Autodesk Inventor part; units mm, degrees
ref_plane "YZ Plane" through (0, 0, 0) normal (1, 0, 0) x (0, 1, 0)
ref_plane "XZ Plane" through (0, 0, 0) normal (0, 1, 0) x (-1, 0, 0)
ref_plane "XY Plane" through (0, 0, 0) normal (0, 0, 1) x (1, 0, 0)
sketch "Sketch1" plane through (0, 0, 0) normal (0, 1, 0) x (-1, 0, 0)
  circle A0 centre (0, 0) radius 73.025
  line L0 (0, 0) -> (0, -73.025) construction
  line L1 (0, 0) -> (-12.6807, -71.9156)
  line L2 (0, 0) -> (12.6807, -71.9156)
  line L3 (0, 0) -> (72.3143, -10.1631)
  line L4 (0, 0) -> (64.4772, -34.2832)
  line L5 (0, 0) -> (32.0121, 65.6344)
  line L6 (0, 0) -> (52.5298, 50.7274)
  line L7 (0, 0) -> (-52.5298, 50.7274)
  line L8 (0, 0) -> (-32.0121, 65.6344)
  line L9 (0, 0) -> (-64.4772, -34.2832)
  line L10 (0, 0) -> (-72.3143, -10.1631)
  circle A1 centre (0, 0) radius 69.85
  arc A2 (4.7597, -69.6876) -> (-4.7597, -69.6876) centre (0, -69.85) ccw
  arc A3 (67.7477, -17.0079) -> (64.806, -26.0614) centre (66.4313, -21.5848) ccw
  arc A4 (37.1107, 59.1762) -> (44.8121, 53.5808) centre (41.0568, 56.5098) ccw
  arc A5 (-44.8121, 53.5808) -> (-37.1107, 59.1762) centre (-41.0568, 56.5098) ccw
  arc A6 (-64.806, -26.0614) -> (-67.7477, -17.0079) centre (-66.4313, -21.5848) ccw
  point P0 (61.6739, -32.7926)
  point P1 (69.1702, -9.7212)
  point P2 (50.2459, 48.5219)
  point P3 (30.6202, 62.7808)
  point P4 (-30.6202, 62.7808)
  point P5 (-50.2459, 48.5219)
  point P6 (-69.1702, -9.7212)
  point P7 (-61.6739, -32.7926)
  point P8 (-12.1293, -68.7888)
  point P9 (12.1293, -68.7888)
  point P10 (64.806, -26.0614)
  point P11 (67.7477, -17.0079)
  point P12 (44.8121, 53.5808)
  point P13 (37.1107, 59.1762)
  point P14 (-37.1107, 59.1762)
  point P15 (-67.7477, -17.0079)
  dimension "d0" = 146.05
  dimension "d1" = 10
  dimension "d4" = 360
  dimension "d6" = 3.175
  dimension "d10" = 9.525
  dimension "d13" = 360
extrude "Extrusion1" add sketch "Sketch1" along normal blind 3.175 contours A0 L3 A1 L6 | L5 A1 L8 A0 | A1 L3 L6 | L6 L5 A1 A4 | A0 L2 A1 L4 | A1 A3 L4 L3 | L5 L8 A1 | L2 A1 A2 L1 | L4 A1 L2 | L10 A1 L7 | L7 A1 A5 L8 | L1 A1 L9 | L9 A1 A6 L10 | A0 L1 A1 L2 | L7 A1 L10 A0 | L1 A0 L9 A1 | A2 A1
fillet "Fillet1" radius 1.5875 24 edges at (30.6202, 1.5875, 62.7808) (32.0121, 1.5875, 65.6344) (-30.6202, 1.5875, 62.7808) (-32.0121, 1.5875, 65.6344) (-52.5298, 1.5875, 50.7274) (-50.2459, 1.5875, 48.5219) (52.5298, 1.5875, 50.7274) (50.2459, 1.5875, 48.5219) (64.4772, 1.5875, -34.2832) (61.6739, 1.5875, -32.7926) (72.3143, 1.5875, -10.1631) (69.1702, 1.5875, -9.7212) (-72.3143, 1.5875, -10.1631) (-69.1702, 1.5875, -9.7212) (-64.4772, 1.5875, -34.2832) (-61.6739, 1.5875, -32.7926) (37.1107, 1.5875, 59.1762) (44.8121, 1.5875, 53.5808) (-44.8121, 1.5875, 53.5808) (-37.1107, 1.5875, 59.1762) (-64.806, 1.5875, -26.0614) (-67.7477, 1.5875, -17.0079) (67.7477, 1.5875, -17.0079) (64.806, 1.5875, -26.0614)
sketch "Sketch5" plane through (0, 3.175, 0) normal (0, 1, 0) x (1, 0, 0)
  line L0 (0, 0) -> (0, 65.0875) construction
  circle A0 centre (0, 50.8) radius 22.225 construction
  arc A1 (63.6995, 35.7075) -> (-63.6995, 35.7075) centre (0, 0) ccw
  circle A2 centre (0, 50.8) radius 12.5 construction
  circle A3 centre (-24.6062, 60.325) radius 1.7526
  circle A4 centre (-24.6062, 60.325) radius 3.175 construction
  circle A5 centre (-22.225, 34.925) radius 3.175 construction
  circle A6 centre (-22.225, 34.925) radius 1.7526
  circle A7 centre (24.6062, 60.325) radius 1.7526 construction
  circle A8 centre (24.6062, 60.325) radius 3.175 construction
  circle A9 centre (22.225, 34.925) radius 3.175 construction
  circle A10 centre (22.225, 34.925) radius 1.7526 construction
  arc A11 (-62.3874, 31.414) -> (-64.248, 27.4085) centre (0, 0) ccw
  arc A12 (63.6995, 35.7075) -> (-63.6995, 35.7075) centre (0, 0) ccw
  line L1 (-28.4451, 67.2572) -> (-25.3861, 34.6286) construction
  line L2 (-22.7046, 31.7864) -> (-3.3572, 28.83) construction
  line L3 (28.4451, 67.2572) -> (25.3861, 34.6286) construction
  line L4 (22.7046, 31.7864) -> (3.3572, 28.83) construction
  circle A13 centre (0, 50.8) radius 6.35 construction
  circle A14 centre (0, 0) radius 73.025
  line L5 (0, 50.8) -> (-8.8388, 59.6388) construction
  circle A15 centre (0, 50.8) radius 9.5 construction
  line L6 (0, 50.8) -> (6.7175, 57.5175) construction
  circle A16 centre (-8.8388, 59.6388) radius 1.5 construction
  circle A17 centre (6.7175, 57.5175) radius 1.5 construction
  circle A18 centre (8.8388, 41.9612) radius 1.5 construction
  circle A19 centre (-6.7175, 44.0825) radius 1.5 construction
  line L7 (-24.6062, 60.325) -> (-22.225, 34.925) construction
  line L8 (-27.7674, 60.0286) -> (-25.3861, 34.6286)
  line L9 (-19.0639, 35.2214) -> (-21.4451, 60.6214)
  arc A20 (-21.4451, 60.6214) -> (-27.7674, 60.0286) centre (-24.6062, 60.325) ccw
  arc A21 (-25.3861, 34.6286) -> (-19.0639, 35.2214) centre (-22.225, 34.925) ccw
  circle A22 centre (-22.225, 34.925) radius 4.7625 construction
  circle A23 centre (-24.6062, 60.325) radius 4.7625 construction
  line L10 (-21.7805, 30.1833) -> (-25.0508, 65.0667) construction
  line L11 (-18.6193, 30.4796) -> (-21.8896, 65.3631)
  line L12 (-28.2119, 64.7704) -> (-24.9416, 29.8869)
  arc A24 (-24.9416, 29.8869) -> (-18.6193, 30.4796) centre (-21.7805, 30.1833) ccw
  arc A25 (-21.8896, 65.3631) -> (-28.2119, 64.7704) centre (-25.0508, 65.0667) ccw
  point P0 (-63.6995, 35.7075)
  point P1 (-23.4156, 47.625)
  point P2 (-63.6995, 35.7075)
  point P3 (-23.4156, 47.625)
  point P4 (-28.3025, 67.3173)
  point P5 (-23.3151, 69.203)
  dimension "d39" = 25
  dimension "d40" = 44.45
  dimension "d78" = 19
  dimension "d100" = 9.525
  dimension "d101" = 9.525
  dimension "d41" = 3.5052
  dimension "d42" = 6.35
  dimension "d43" = 9.525
  dimension "d44" = 24.6062
  dimension "d45" = 6.35
  dimension "d46" = 3.5052
  dimension "d47" = 15.875
  dimension "d48" = 22.225
  dimension "d68" = 12.7
  dimension "d77" = 315
  dimension "d79" = 3
  dimension "d80" = 3
  dimension "d83" = 360
  dimension "d102" = 6.35
extrude "Extrusion3" cut sketch "Sketch5" against normal blind 25.4
chamfer "Chamfer2" distance 1.524 angle 41 2 edges at (-23.9776, 3.175, -34.925) (-26.3589, 3.175, -60.325)
equation "\"d45\" = d42"
equation "\"d46\" = d41"
properties part number "Top Plate" material "UHMW, White"
Read the model definition and answer for the solid it produces. Units are mm, in the model's axes. Give positions to 0.01 mm unless a question says otherwise; leave off trailing zeros. Write each loop counter-clockwise with the first axis right and the second up, starting at its lowest first coordinate (ties: lowest second). Pieces come first, ordered by that corner, then holes. Notation, with made-up numbers: (58.25, -24.75) -> (88.25, -24.75) arc R23 ccw to (88.25, -15.75) -> close; hole circle Ø10 at (52.5, -10.75). An arc over 180 degrees is marked (long way). Answer in a Markdown table with one row per item.
1) This flat-tipped pin is pushed along its axis until it touches: pin 1 Ø5.5 at (x, z) = (-22.225, -34.925) entering from -Y. Where does it stop, or does it pass through?
Results list:
| item | result |
|---|---|
| pin 1 | y = 0 |
2) Section B-B on z = -44 is taken. Give the vertices of the cut face in (x, y) (3 decimals), plus the area to 3 significant figures.
Results list:
| item | result |
|---|---|
| outline | (-26.265, 0) -> (-19.887, 0) -> (-19.887, 3.175) -> (-26.265, 3.175) -> close |
| area | 20.2 mm^2 |
3) Straight lines are drawn through the part: line 1 (Z direction, x = -23.25, y = 1.55); line 2 (Z direction, x = -23.5, y = 1.6); line 3 (Z direction, x = -24.25, y = 0.4). For each, find the intervals that lie inside material, in ascending order. Write a range as [from, to].
Results list:
| item | result |
|---|---|
| line 1 | [-67.68, -61.44], [-59.21, -36.35], [-33.5, -27.37] |
| line 2 | [-67.84, -61.68], [-58.97, -36.13], [-33.72, -27.51] |
| line 3 | [-68.14, -62.04], [-58.61, -28.19] |
4) Determine the mould class of faces 1 (the cylindrical face through (-20.606, 0.938, -34.254)), 2 (the cylindrical face through (-23.8, 0.94, -58.77)), 3 (the flat face through (-22, 3.175, -30)), 4 (the cylindrical face through (-21.554, 1.61, -27.016)) for opening direction X: released by +X, released by -X, zero draft, split by the parting line, or undercut.
Results list:
| item | result |
|---|---|
| face 1 | undercut |
| face 2 | undercut |
| face 3 | zero draft |
| face 4 | split by the parting line |
5) Section A-A on y = 1.4 is taken. Give the vertices of the cut face in (x, z) (3 decimals).
Results list:
| item | result |
|---|---|
| outline | (-28.212, -64.77) arc R3.175 ccw to (-21.89, -65.363) -> (-21.445, -60.621) -> (-19.064, -35.221) -> (-18.619, -30.48) arc R3.175 ccw to (-24.942, -29.887) -> (-25.386, -34.629) -> (-27.767, -60.029) -> close; hole circle Ø3.505 at (-24.606, -60.325); hole circle Ø3.505 at (-22.225, -34.925) |
